The model under review builds one solid part; all positions refer to its coordinate system, in mm. A direction names the side the tool comes from. Give positions to 0.01 mm unless a question says otherwise; leave off trailing zeros. Loops run counter-clockwise (first coordinate to the right, second up) from the corner with the lowest first, then second, coordinate; pieces in that order, holes last. Notation, with made-up numbers: M -19.5,71 L -4.5,71 A14 ccw -4.5,97 Z; hole C -10.75,46.25 d2. An arc over 180 degrees is marked long. Return JSON: item names as keys, results as strings.
```python
from build123d import *

# Parameters (mm, degrees)
F0_W     = 90
F0_H     = 20
F0_W_2   = 10
F1_DEPTH = 52
F3_D     = 20
F5_D     = 20
F6_R     = 25.99999
F7_DEPTH = 312


# Not quite as in the source:
# - a fillet or chamfer is up to 0.001 mm smaller than in the source, because OpenCascade refuses the exact size


with BuildPart() as f1:
    # F0 (on Front) → F1 (new body)
    with BuildSketch(Plane.XZ):
        Polygon((-16.9582804857, -1.5154299321), (-16.9582804857, 18.4845700679), (-28.6740092382, 18.4845700679), (-68.0709788579, 57.8815396876), (-82.2131144816, 72.0236753113), (-93.5268229806, 83.3373838103), (-107.6689586043, 69.1952481866), (-36.9582804857, -1.5154299321), align=None)
        with Locations((28.0417195143, 8.4845700679)):
            Rectangle(F0_W, F0_H)
        with Locations((78.0417195143, 8.4845700679)):
            Rectangle(F0_W_2, F0_H)
    extrude(amount=F1_DEPTH)

    # F3 (through all)
    with Locations(Plane.XY.offset(18.4845700679)):
        with Locations((63.4629929066, -26), (-6.8132670224, -26)):
            Hole(F3_D / 2)

    # F5 (through all)
    with Locations(Plane(origin=(-5.0947195851, 0, -5.0947195851), x_dir=(0, 1, 0), z_dir=(0.7071067812, 0, 0.7071067812))):
        with Locations((-26, 99.061879971)):
            Hole(F5_D / 2)

    # F6 (radius 26 in the source; OpenCascade refuses exactly that, so slightly less here)
    f6_edges = [f1.edges().sort_by_distance(p)[0] for p in [
        (-100.597891, 0, 76.266316),
        (-100.597891, -52, 76.266316),
    ]]
    fillet(f6_edges, radius=F6_R)

    # F2 (on face) → F7 (cut)
    with BuildSketch(Plane.XY.offset(18.4845700679)):
        Polygon((63.1867329776, -36), (63.1867329776, -26), (52.6720061898, -26), (0, -26), (-5.5663499609, -26), (-6.8132670224, -26), (-6.8132670224, -36), align=None)
        Polygon((52.6720061898, -26), (63.1867329776, -26), (63.1867329776, -16), (-6.8132670224, -16), (-6.8132670224, -26), (-5.5663499609, -26), (0, -26), align=None)
    extrude(amount=-F7_DEPTH, mode=Mode.SUBTRACT)


solid = f1.part
```
1) Insertion check: pin 1 (5 mm diameter, centred on y = -40, z = 36.5, fed in from -X); pin 2 (3 mm diameter, centred on x = 20, y = -35, fed in from +Z); pin 3 (8 mm diameter, centred on x = -81, y = -16.5, fed in from -Z). Each pin has a flat end and moves straight along its axis. Give the tip position at first contact, or say it passes through.
From the geometry:
{"pin 1": "x = -77.47", "pin 2": "z = 18.48", "pin 3": "z = 38.53"}
2) Wall thickness on L1, parallel to Y at x = 36.5, z = 8; L2, parallel to Z at x = 49.5, y = -37.5; L3, parallel to X at y = -47, z = 13.5: over which ranges is each line inside the solid? List them lowest first. Write a range as from..to.
From the geometry:
{"L1": "-52..-36, -16..0", "L2": "-1.52..18.48", "L3": "-51.97..83.04"}
3) Consider section A-A on x = -0.5. Write out the cut boundary in (y, z).
From the geometry:
{"outline": "M -52,-1.52 L -36,-1.52 L -36,18.48 L -52,18.48 Z; M -16,-1.52 L 0,-1.52 L 0,18.48 L -16,18.48 Z"}
4) Consider section C-C on x = -26. Write out the cut boundary in (y, z).
From the geometry:
{"outline": "M -52,-1.52 L 0,-1.52 L 0,18.48 L -52,18.48 Z"}
5) Consider section D-D on y = -9. Write out the cut boundary in (x, z).
From the geometry:
{"outline": "M -103.19,64.72 L -36.96,-1.52 L 83.04,-1.52 L 83.04,18.48 L -28.67,18.48 L -89.05,78.86 Z"}
6) The part is to be moulded in two halves that separate along X. For faces 4 (the face through (29, -16, 9)), 5 (the face through (22, -14, -1.515)), 6 (the face through (-95.168, -44.586, 70.639)), say which applies: released by +X, released by -X, zero draft, split by the parting line, or undercut.
From the geometry:
{"face 4": "undercut", "face 5": "zero draft", "face 6": "released by -X"}
7) Consider section B-B on y = -21. Write out the cut boundary in (x, z), then the cut area to 3 significant figures.
From the geometry:
{"outline": "M -107.33,68.85 L -95.41,56.93 L -81.27,71.08 L -93.18,82.99 Z; M -83.16,44.69 L -36.96,-1.52 L -15.47,-1.52 L -15.47,18.48 L -28.67,18.48 L -69.02,58.83 Z; M 72.12,-1.52 L 83.04,-1.52 L 83.04,18.48 L 72.12,18.48 Z", "area": "2,130 mm²"}
8) Tool access review of faces 1 (the face through (-10, 0, 15)), 2 (the face through (28, -14, 18.485)), 3 (the face through (-16.81, -26.22, 8.34)): name each direction out of +Z, -Z, +X, -X, +Y, -Y from which nothing blocks a thin tool from reaching the whole face with its end or side.
From the geometry:
{"face 1": "+Z, -Z, +X, -X, +Y", "face 2": "+Z, +X, +Y, -Y", "face 3": "+Z, -Z"}
